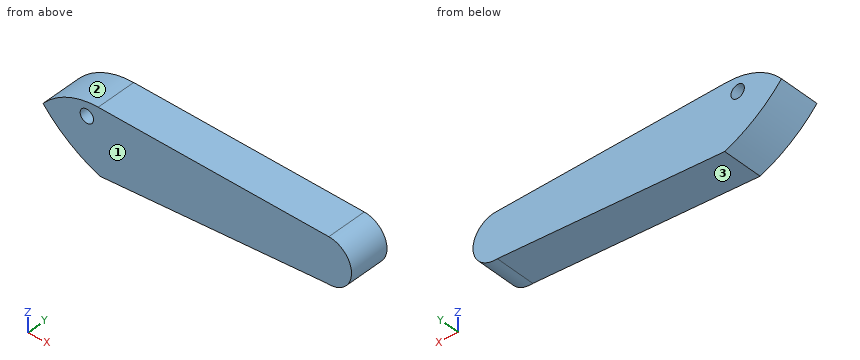
from build123d import *

# Parameters (mm, degrees)
F0_R     = 2.582307
F1_DEPTH = 15.24


with BuildPart() as f1:
    # F0 (on Front) → F1 (new body)
    with BuildSketch(Plane.XZ):
        with BuildLine():
            Line((35.072878, 13.622056), (-53.861916, 13.622056))
            ThreePointArc((-53.861916, 13.622056), (-65.629053, 10.991668), (-75.156167, 3.601233))
            ThreePointArc((-75.156167, 3.601233), (-65.141959, -5.294066), (-53.235617, -11.430001))
            Line((-53.235617, -11.430001), (34.446575, -3.914384))
            ThreePointArc((34.446575, -3.914384), (43.846688, 4.529301), (35.072878, 13.622056))
        make_face()
        with Locations((-58.246028, 7.985342)):
            Circle(F0_R, mode=Mode.SUBTRACT)
    extrude(amount=F1_DEPTH)


solid = f1.part
Input: part model. Units: mm. Frame: model coordinates. Face numbers are marked on the shaded views. Coordinates: 2 decimals unless noted, no trailing zeros. Order: outer loops, then holes, each group sorted by start corner. A loop starts at its lowest first (then second) coordinate and runs counter-clockwise, first axis right, second up. Notation, with made-up numbers: M 75.25,-1 L 107.25,-1 A26 cw 107.25,23 Z; hole C 23,44 d6. An arc over 180 degrees is marked long. One line per question, with ' | ' between items.
Item 1: Section B-B (y = -6). Output: boundary loops of the cut face in (x, z).
Geometry results:
outline: M -75.16,3.6 A53.62 ccw -53.24,-11.43 L 34.45,-3.91 A8.78 ccw long 35.07,13.62 L -53.86,13.62 A27.64 ccw Z; hole C -58.25,7.99 d5.16
Item 2: Draft query along X for the marked faces 1, 2 and 3. Return one class per face: released by +X, released by -X, zero draft, split by the parting line, or undercut.
Geometry results:
face 1: zero draft | face 2: released by -X | face 3: released by +X
Item 3: Pin query (flat end, axial travel): pin 1 (5 mm diameter, centred on y = -2, z = -5, fed in from +X); pin 2 (4 mm diameter, centred on y = -12, z = -1, fed in from -X); pin 3 (2 mm diameter, centred on x = -32, z = 7.5, fed in from +Y); pin 4 (3 mm diameter, centred on y = -12, z = 1.5, fed in from +X). Return the tip coordinate at first contact, or that it passes through.
Geometry results:
pin 1: stops at x = 39.89 | pin 2: stops at x = -72.72 | pin 3: stops at y = 0 | pin 4: stops at x = 43.66
Item 4: Ray query, line 1 along X through (y, z) = (-1.5, 7); line 2 along Z through (x, y) = (29.5, -4.5); line 3 along X through (y, z) = (-13.5, -1.25). Return the intervals inside material, ascending.
Geometry results:
line 1: x = -71.81 to -60.63, -55.86 to 43.58 | line 2: z = -4.34 to 13.62 | line 3: x = -70.33 to 41.39
Item 5: Section A-A (z = 9.25). Output: boundary loops of the cut face in (x, y), then the cut area to 3 significant figures.
Geometry results:
outline: M -68.78,-15.24 L -60.5,-15.24 L -60.5,0 L -68.78,0 Z; M -55.99,-15.24 L 42.67,-15.24 L 42.67,0 L -55.99,0 Z | area: 1,630 mm^2
Item 6: Section D-D (x = -48). Output: boundary loops of the cut face in (y, z).
Geometry results:
outline: M -15.24,-10.98 L 0,-10.98 L 0,13.62 L -15.24,13.62 Z
Item 7: Section C-C (z = -7.25). Output: boundary loops of the cut face in (x, y).
Geometry results:
outline: M -62.07,-15.24 L -4.47,-15.24 L -4.47,0 L -62.07,0 Z
